```python
from build123d import *

# Parameters (mm, degrees)
F1_DEPTH  = 79
F2_W      = 106
F2_H      = 2
F3_DEPTH  = 48
F4_W      = 10
F4_H      = 20
F5_DEPTH  = 150
F6_W      = 59.092542
F6_H      = 51.87012
F7_DEPTH  = 2
F8_R      = 1.75
F9_DEPTH  = 25
F11_DEPTH = 1.5


with BuildPart() as f1:
    # F0 (on Top) → F1 (new body)
    with BuildSketch(Plane.XY):
        Polygon((0, 110), (-50, 110), (-50, 108), (-2, 108), (-2, 2), (-50, 2), (-50, 0), (0, 0), align=None)
    extrude(amount=F1_DEPTH)

    # F2 (on face) → F3 (join)
    with BuildSketch(Plane(origin=(-2, 0, 0), x_dir=(0, -1, 0), z_dir=(-1, 0, 0))):
        with Locations((-55, 1)):
            Rectangle(F2_W, F2_H)
    extrude(amount=F3_DEPTH)

    # F4 (on face) → F5 (cut)
    with BuildSketch(Plane.XZ):
        with Locations((-45, 69)):
            Rectangle(F4_W, F4_H)
    extrude(amount=-F5_DEPTH, mode=Mode.SUBTRACT)

    # F6 (on face) → F7 (join)
    with BuildSketch(Plane(origin=(-2, 0, 0), x_dir=(0, -1, 0), z_dir=(-1, 0, 0))):
        with Locations((-44.822951, 35.747332)):
            Rectangle(F6_W, F6_H)
    extrude(amount=F7_DEPTH)

    # F8 (on face) → F9 (cut)
    with BuildSketch(Plane.YZ):
        Polygon((61.5, 50), (20, 50), (20, 20), (61.5, 20), (68, 26.5), (68, 43.5), align=None)
        with Locations((44, 55)):
            Circle(F8_R)
        with Locations((44, 15)):
            Circle(F8_R)
    extrude(amount=-F9_DEPTH, mode=Mode.SUBTRACT)

    # F10 (on face) → F11 (join)
    with BuildSketch(Plane.XZ):
        with BuildLine():
            Line((-37, 62), (-12, 62))
            ThreePointArc((-12, 62), (-10.75, 63.25), (-12, 64.5))
            Line((-12, 64.5), (-37, 64.5))
            ThreePointArc((-37, 64.5), (-38.25, 63.25), (-37, 62))
        make_face()
    extrude(amount=F11_DEPTH)


solid = f1.part
```
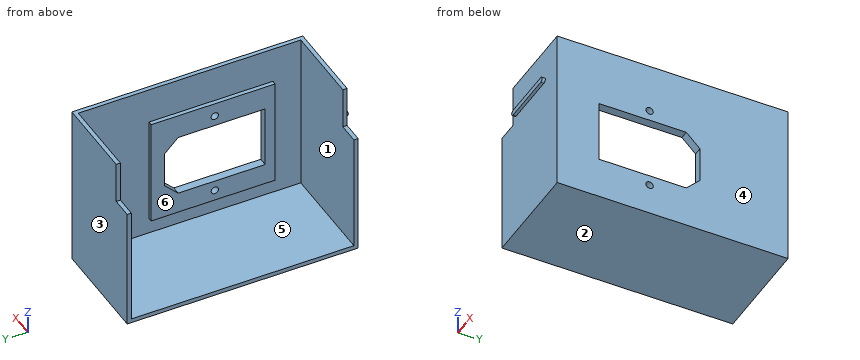
Check sheet for the modelled part. Datum: model origin and axes. Units: mm. Face numbers are marked on the shaded views. A direction names the side the tool comes from. Round coordinates to 2 decimals unless told otherwise and drop trailing zeros. Loops run counter-clockwise (first coordinate to the right, second up) from the corner with the lowest first, then second, coordinate; pieces in that order, holes last. Notation, with made-up numbers: (-29.75, -35) - (15.25, -35) arc R36 ccw to (15.25, 1) - close; hole circle Ø8 at (73, 31). An arc over 180 degrees is marked (long way). Write item = value, one per line. Start each with the question number.
Q1. Release check for a two-part mould opening along Y. For the marked faces 3, 4, 5 and 6 record: pulls with the +Y half, pulls with the -Y half, needs draft (parallel to the pull), parting line crosses it, or undercut.
Q2. Section check D-D (z = 63.25). Record the boundary of the cut face in (x, y).
Q3. Thickness scan on L1, parallel to Z at x = -0.85, y = 44; L2, parallel to Y at x = -22, z = 29; L3, parallel to Z at x = -3, y = 44. Record the ranges inside material, lowest first.
Q4. Depth check by flat-ended pin: P1, Ø1, axis at x = -38, z = 20, coming from the -Y side; P2, Ø4.5, axis at y = 44, z = 55, coming from the -X side; P3, Ø0.6, axis at x = -44, y = 1.5, coming from the +Z side; P4, Ø23, axis at y = 33.5, z = 35.5, coming from the -X side. Enter the tip coordinate at first touch or a pass-through.
Q5. Section check C-C (y = 60). Record the boundary of the cut face in (x, z), plus the area to 3 significant figures.
Q6. Section check A-A (y = 44). Record the boundary of the cut face in (x, z).
Q7. Access from +Z, -Z, +X, -X, +Y, -Y to the whole of each face (thin tool, end or side, straight path). Record for the marked faces 1 and 2.
Q8. Section check B-B (z = 55). Record the boundary of the cut face in (x, y), plus the area to 3 significant figures.
Derived:
q1.face_3 = pulls with the +Y half
q1.face_4 = needs draft
q1.face_5 = undercut
q1.face_6 = undercut
q2.outline = (-40, 0) - (-38.25, 0) - (-38.25, -1.5) - (-10.75, -1.5) - (-10.75, 0) - (0, 0) - (0, 110) - (-40, 110) - (-40, 108) - (-2, 108) - (-2, 2) - (-40, 2) - close
q3.L1 = 0 to 13.25, 16.75 to 20, 50 to 53.25, 56.75 to 79
q3.L2 = 0 to 2, 108 to 110
q3.L3 = 0 to 2, 9.81 to 13.25, 16.75 to 20, 50 to 53.25, 56.75 to 61.68
q4.P1 = 0
q4.P2 = -4
q4.P3 = 59
q4.P4 = through
q5.outline = (-50, 0) - (0, 0) - (0, 20) - (-4, 20) - (-4, 9.81) - (-2, 9.81) - (-2, 2) - (-50, 2) - close; (-4, 50) - (0, 50) - (0, 79) - (-2, 79) - (-2, 61.68) - (-4, 61.68) - close
q5.area = 238 mm^2
q6.outline = (-50, 0) - (0, 0) - (0, 13.25) - (-4, 13.25) - (-4, 9.81) - (-2, 9.81) - (-2, 2) - (-50, 2) - close; (-4, 16.75) - (0, 16.75) - (0, 20) - (-4, 20) - close; (-4, 50) - (0, 50) - (0, 53.25) - (-4, 53.25) - close; (-4, 56.75) - (0, 56.75) - (0, 79) - (-2, 79) - (-2, 61.68) - (-4, 61.68) - close
q7.face_1 = +Z, -X
q7.face_2 = -Z, +X, -X, +Y, -Y
q8.outline = (-50, 0) - (0, 0) - (0, 42.25) - (-4, 42.25) - (-4, 15.28) - (-2, 15.28) - (-2, 2) - (-50, 2) - close; (-50, 108) - (-2, 108) - (-2, 74.37) - (-4, 74.37) - (-4, 45.75) - (0, 45.75) - (0, 110) - (-50, 110) - close
q8.area = 516 mm^2
